Source: CAD feature listing. Evaluate the final solid. Frame: model axes, mm. A direction names the side the tool comes from. Coordinates: 2 decimals unless noted, no trailing zeros. Loops run counter-clockwise (first coordinate to the right, second up) from the corner with the lowest first, then second, coordinate; pieces in that order, holes last. Notation, with made-up numbers: (-14, -36.5) - (26, -36.5) arc R18 ccw to (26, -13.5) - close; hole circle Ø10 at (-24.5, -16.5). An arc over 180 degrees is marked (long way). Write item = value, one per line. Start each with the question number.
Autodesk Inventor part; units mm, degrees
ref_plane "YZ Plane" through (0, 0, 0) normal (1, 0, 0) x (0, 1, 0)
ref_plane "XZ Plane" through (0, 0, 0) normal (0, 1, 0) x (-1, 0, 0)
ref_plane "XY Plane" through (0, 0, 0) normal (0, 0, 1) x (1, 0, 0)
sketch "Sketch1" plane through (0, 0, 0) normal (0, 0, 1) x (1, 0, 0)
  circle A0 centre (0, 0) radius 95
  circle A1 centre (-56.5685, 56.5685) radius 8.5
  circle A2 centre (0, 0) radius 80 construction
  circle A3 centre (-56.5685, -56.5685) radius 8.5
  circle A4 centre (56.5685, -56.5685) radius 8.5
  circle A5 centre (56.5685, 56.5685) radius 8.5
  line L0 (17.8112, -43) -> (-17.8112, -43)
  line L1 (-17.8112, -43) -> (-43, -17.8112)
  line L2 (-43, -17.8112) -> (-43, 17.8112)
  line L3 (-43, 17.8112) -> (-17.8112, 43)
  line L4 (-17.8112, 43) -> (17.8112, 43)
  line L5 (17.8112, 43) -> (43, 17.8112)
  line L6 (43, 17.8112) -> (43, -17.8112)
  line L7 (43, -17.8112) -> (17.8112, -43)
  line L8 (0, 0) -> (-30.4056, 30.4056) construction
  dimension "d171" = 160
  dimension "d157" = 190
  dimension "d170" = 17
  dimension "d174" = 360
  dimension "d176" = 86
extrude "Plate5" add sketch "Sketch1" along normal blind 3
properties part number "PRS 9651 DrSysB MAIN  FLANGE_D1200" material "Stainless Steel"
Item 1: Material intervals for L1, parallel to Y at x = -4.5, z = 1.5; L2, parallel to X at y = -2, z = 0.75; L3, parallel to X at y = 32, z = 1.2, sorted ascending. Write a range as [from, to].
Item 2: Cut plane D-D (x = -56). Return the cut outline in (y, z).
Item 3: Reachability of faces 4 (the flat face through (-1, 44, 3)), 5 (the flat face through (30.58, -30.23, 1.48)) from +Z, -Z, +X, -X, +Y, -Y: full face, straight path, thin tool, end or side. Return the list, or none.
Item 4: First-contact query: pin 1 (8 mm diameter, centred on x = 37.5, y = -12, fed in from -Z); pin 2 (22 mm diameter, centred on x = -56.57, y = -56.57, fed in from -Z); pin 3 (1.5 mm diameter, centred on x = 8.5, z = 1, fed in from -Y); pin 4 (1 mm diameter, centred on y = 16, z = 1.5, fed in from -X). Flat tips, straight axial feed; report the tip coordinate or a pass-through.
Item 5: Cut plane C-C (z = 1.25). Return the cut outline in (x, y).
Item 6: Cut plane A-A (y = 0). Return the cut outline in (x, z).
Item 7: Draft query along Y for faces 1 (the cylindrical face through (-51.999, -63.736, 1.479)), 2 (the cylindrical face through (-20.59, 92.74, 1.48)), 3 (the flat face through (-1, 44, 0)). Return one class per face: released by +Y, released by -Y, zero draft, split by the parting line, or undercut.
Responses:
q1.L1 = [-94.89, -43], [43, 94.89]
q1.L2 = [-94.98, -43], [43, 94.98]
q1.L3 = [-89.45, -28.81], [28.81, 89.45]
q2.outline = (-76.74, 0) - (-65.05, 0) - (-65.05, 3) - (-76.74, 3) - close; (-48.09, 0) - (48.09, 0) - (48.09, 3) - (-48.09, 3) - close; (65.05, 0) - (76.74, 0) - (76.74, 3) - (65.05, 3) - close
q3.face_4 = +Z, +X, -X, +Y, -Y
q3.face_5 = +Z, -Z
q4.pin_1 = through
q4.pin_2 = 0
q4.pin_3 = -94.68
q4.pin_4 = -93.73
q5.outline = circle Ø190 at (0, 0); hole circle Ø17 at (-56.57, -56.57); hole circle Ø17 at (-56.57, 56.57); hole (-43, -17.81) - (-17.81, -43) - (17.81, -43) - (43, -17.81) - (43, 17.81) - (17.81, 43) - (-17.81, 43) - (-43, 17.81) - close; hole circle Ø17 at (56.57, -56.57); hole circle Ø17 at (56.57, 56.57)
q6.outline = (-95, 0) - (-43, 0) - (-43, 3) - (-95, 3) - close; (43, 0) - (95, 0) - (95, 3) - (43, 3) - close
q7.face_1 = undercut
q7.face_2 = split by the parting line
q7.face_3 = zero draft
